Part model, mm, in its own coordinate system. A direction names the side the tool comes from. Round coordinates to 2 decimals unless told otherwise and drop trailing zeros. Order: outer loops, then holes, each group sorted by start corner. A loop starts at its lowest first (then second) coordinate and runs counter-clockwise, first axis right, second up. Notation, with made-up numbers: (84, 28.5) - (125, 28.5) arc R19 ccw to (125, 35.5) - close; hole circle Ø5 at (-37, -29). An arc over 180 degrees is marked (long way). Answer as a JSON object with one key per item and string values.
```python
from build123d import *

# Parameters (mm, degrees)
BOSS_EXTRUDE1_DEPTH      = 10
BOSS_EXTRUDE1_DEPTH_BACK = 10
SKETCH1_R                = 1.5
CUT_EXTRUDE1_DEPTH       = 15.053645347
CUT_EXTRUDE1_DEPTH_BACK  = 15.053645347
SKETCH2_W                = 9.15922742
SKETCH2_H                = 4
FILLET1_R                = 3
BOSS_EXTRUDE2_START      = 22
BOSS_EXTRUDE2_DEPTH      = 22
CUT_EXTRUDE2_DEPTH       = 15
CUT_EXTRUDE3_DEPTH       = 15
SKETCH7_R                = 1.5
BOSS_EXTRUDE3_DEPTH      = 17


with BuildPart() as part:
    # Sketch1 → Boss-Extrude1 (new, two sides: drawn at the far end of the back side and taken through both)
    with BuildSketch(Plane(origin=(0, 0, 0), x_dir=(1, 0, 0), z_dir=(0, 1, 0)).offset(-BOSS_EXTRUDE1_DEPTH_BACK)):
        with BuildLine():
            Line((-5, -8.514983708), (5, -8.514983708))
            Line((5, -8.514983708), (5, 0))
            ThreePointArc((5, 0), (0, 5), (-5, 0))
            Line((-5, 0), (-5, -8.514983708))
        make_face()
        with Locations(Location((0, 0, 0), (0, 0, 270))):
            Circle(SKETCH1_R, mode=Mode.SUBTRACT)
    extrude(amount=BOSS_EXTRUDE1_DEPTH + BOSS_EXTRUDE1_DEPTH_BACK)

    # Sketch2 → Cut-Extrude1 (cut, two sides: drawn at the far end of the back side and taken through both)
    with BuildSketch(Plane(origin=(0, 0, 0), x_dir=(0, 0, -1), z_dir=(1, 0, 0)).offset(-CUT_EXTRUDE1_DEPTH_BACK)):
        with Locations((0.42038629, 6)):
            Rectangle(SKETCH2_W, SKETCH2_H)
        with Locations((0.42038629, 0.5)):
            Rectangle(SKETCH2_W, SKETCH2_H)
        with Locations((0.42038629, -5)):
            Rectangle(SKETCH2_W, SKETCH2_H)
    extrude(amount=CUT_EXTRUDE1_DEPTH + CUT_EXTRUDE1_DEPTH_BACK, mode=Mode.SUBTRACT)

    # Fillet1
    fillet1_edges = [part.edges().sort_by_distance(p)[0] for p in [
        (0, -10, 8.514983708),
        (0, 10, 8.514983708),
    ]]
    fillet(fillet1_edges, radius=FILLET1_R)

    # Sketch3 → Boss-Extrude2 (add)
    with BuildSketch(Plane(origin=(5, 0, 0), x_dir=(0, 0, -1), z_dir=(1, 0, 0)).offset(BOSS_EXTRUDE2_START)):
        with BuildLine():
            Line((-4.15922742, 8), (-6.514983708, 8))
            Line((-6.514983708, 8), (-6.514983708, -7))
            Line((-6.514983708, -7), (-4.15922742, -7))
            Line((-4.15922742, -7), (0, -7))
            Line((0, -7), (0, -10))
            Line((0, -10), (-5.514983708, -10))
            ThreePointArc((-5.514983708, -10), (-7.636304051, -9.121320344), (-8.514983708, -7))
            Line((-8.514983708, -7), (-8.514983708, 7))
            ThreePointArc((-8.514983708, 7), (-7.636304051, 9.121320344), (-5.514983708, 10))
            Line((-5.514983708, 10), (0, 10))
            Line((0, 10), (0, 8))
            Line((0, 8), (-4.15922742, 8))
        make_face()
    extrude(amount=-BOSS_EXTRUDE2_DEPTH)

    # Sketch4 → Cut-Extrude2 (cut)
    with BuildSketch(Plane(origin=(0, 0, 6.514983708), x_dir=(-1, 0, 0), z_dir=(0, 0, -1))):
        with BuildLine():
            ThreePointArc((-9.210889788, 1.490024104), (-21.733598121, 0), (-9.210889788, -1.490024104))
            ThreePointArc((-9.210889788, -1.490024104), (-7.883598121, 0), (-9.210889788, 1.490024104))
        make_face()
    extrude(amount=-CUT_EXTRUDE2_DEPTH, mode=Mode.SUBTRACT)

    # Sketch6 → Cut-Extrude3 (cut)
    with BuildSketch(Plane(origin=(0, 0, 6.514983708), x_dir=(-1, 0, 0), z_dir=(0, 0, -1))):
        Polygon((-22.036773602, 3.704956115), (-28.57394985, 10.876283833), (-25.617841784, 13.570986989), (-19.080665536, 6.399659271), align=None)
    extrude(amount=CUT_EXTRUDE3_DEPTH, mode=Mode.SUBTRACT)

    # Sketch7 → Boss-Extrude3 (add)
    with BuildSketch(Plane.XZ.offset(-8)):
        with Locations(Location((5.358426028, 1.456547556, 0), (0, 0, 256.175382735))):
            Circle(SKETCH7_R)
    extrude(amount=BOSS_EXTRUDE3_DEPTH)


solid = part.part
```
Item 1: Drop flat-ended pins along their axis: P1, Ø1.5, axis at y = 4, z = 5, coming from the +X side; P2, Ø8, axis at x = 8, y = 5.5, coming from the -Z side; P3, Ø1, axis at x = 16.5, y = 9, coming from the -Z side. Give the stop position or say it passes through.
Taken from the geometry:
{"P1": "x = 5", "P2": "z = -2.57", "P3": "z = 0"}
Item 2: Cut at D-D (z = 2). Write the cut outline in (x, y), plus the area to 3 significant figures.
Taken from the geometry:
{"outline": "(-5, -10) - (27, -10) - (27, -7) - (6.76, -7) - (6.76, 8) - (20.54, 8) - (22.36, 10) - (-5, 10) - (-5, 8) - (3.96, 8) - (3.96, 4) - (-5, 4) - (-5, 2.5) - (3.96, 2.5) - (3.96, -1.5) - (-5, -1.5) - (-5, -3) - (3.96, -3) - (3.96, -7) - (-5, -7) - close; (25.95, 8) - (27, 8) - (27, 9.15) - close", "area": "218 mm2"}
Item 3: Two-plate mould, pull along X, no slides. Class faces 4 (the flat face through (-5, 0, 5)), 5 (the flat face through (8, 8, 2)), 6 (the flat face through (21.46, 9.01, 3.3)): pulls with the +X half, pulls with the -X half, needs draft (parallel to the pull), parting line crosses it, or undercut.
Taken from the geometry:
{"face 4": "pulls with the -X half", "face 5": "needs draft", "face 6": "undercut"}
Item 4: Tool access for faces 1 (the flat face through (26.5, 8, 3.2)), 2 (the cylindrical face through (7.884, -0.031, 7.501)), 3 (the flat face through (7.7, -0.1, 8.515)): list every direction of +Z, -Z, +X, -X, +Y, -Y with a clear straight run to the whole face (end or side of a thin tool).
Taken from the geometry:
{"face 1": "-Z, +X", "face 2": "+Z, -Z", "face 3": "+Z, +X, -X, +Y, -Y"}
Item 5: Probe L1, parallel to Z at x = 5.5, y = -3.5; L2, parallel to Y at x = 6, z = 3; L3, parallel to Z at x = 0, y = 0.25. List the from-to ranges inside material, lowest first. Write a range as from..to.
Taken from the geometry:
{"L1": "-0.04..2.95, 6.51..8.51", "L2": "-10..-7, 8..10", "L3": "4.16..8.51"}
Item 6: Cut at B-B (y = 0). Write the cut outline in (x, z).
Taken from the geometry:
{"outline": "(-5, 4.16) - (5, 4.16) - (5, 6.51) - (7.88, 6.51) - (7.88, 8.51) - (-5, 8.51) - close; circle Ø3 at (5.36, 1.46); (21.73, 6.51) - (27, 6.51) - (27, 8.51) - (21.73, 8.51) - close"}
Item 7: Cut at C-C (x = 0). State how many separate pieces and enclosed holes the cut face has, plus the area to 3 significant figures.
Taken from the geometry:
{"separate pieces": "5", "enclosed holes": "0", "area": "133 mm2"}
Item 8: Cut at A-A (z = 3.5). Write the cut outline in (x, y), plus the area to 3 significant figures.
Taken from the geometry:
{"outline": "(-5, -10) - (27, -10) - (27, -7) - (-5, -7) - close; (-5, -3) - (5, -3) - (5, -1.5) - (-5, -1.5) - close; (-5, 2.5) - (5, 2.5) - (5, 4) - (-5, 4) - close; (-5, 8) - (20.54, 8) - (22.36, 10) - (-5, 10) - close; (25.95, 8) - (27, 8) - (27, 9.15) - close", "area": "180 mm2"}
